Source: CAD feature listing. Evaluate the final solid. Frame: model axes, mm. Coordinates: 2 decimals unless noted, no trailing zeros. Order: outer loops, then holes, each group sorted by start corner. A loop starts at its lowest first (then second) coordinate and runs counter-clockwise, first axis right, second up.
```python
from build123d import *

# Parameters (mm, degrees)
BOSS_EXTRUDE1_DEPTH = 10


with BuildPart() as part:
    # Sketch1 → Boss-Extrude1 (new body)
    with BuildSketch(Plane(origin=(0, 0, 0), x_dir=(1, 0, 0), z_dir=(0, 1, 0))):
        with BuildLine():
            ThreePointArc((2.7, 0), (2.693734095, 0.183838592), (2.674965461, 0.366823913))
            Line((2.674965461, 0.366823913), (1.655161558, 2.133176087))
            ThreePointArc((1.655161558, 2.133176087), (1.35, 2.33826859), (1.019803903, 2.5))
            Line((1.019803903, 2.5), (-1.019803903, 2.5))
            ThreePointArc((-1.019803903, 2.5), (-1.35, 2.33826859), (-1.655161558, 2.133176087))
            Line((-1.655161558, 2.133176087), (-2.674965461, 0.366823913))
            ThreePointArc((-2.674965461, 0.366823913), (-2.7, 0), (-2.674965461, -0.366823913))
            Line((-2.674965461, -0.366823913), (-1.655161558, -2.133176087))
            ThreePointArc((-1.655161558, -2.133176087), (-1.35, -2.33826859), (-1.019803903, -2.5))
            Line((-1.019803903, -2.5), (1.019803903, -2.5))
            ThreePointArc((1.019803903, -2.5), (1.35, -2.33826859), (1.655161558, -2.133176087))
            Line((1.655161558, -2.133176087), (2.674965461, -0.366823913))
            ThreePointArc((2.674965461, -0.366823913), (2.693734095, -0.183838592), (2.7, 0))
        make_face()
    extrude(amount=BOSS_EXTRUDE1_DEPTH)


solid = part.part
```
1. Section query A-A on y = 1.5. Return loops of the section in (x, z), plus the area to 3 significant figures.
Findings:
outline: (-2.67, -0.37) - (-1.66, -2.13) arc R2.7 ccw to (-1.02, -2.5) - (1.02, -2.5) arc R2.7 ccw to (1.66, -2.13) - (2.67, -0.37) arc R2.7 ccw to (2.67, 0.37) - (1.66, 2.13) arc R2.7 ccw to (1.02, 2.5) - (-1.02, 2.5) arc R2.7 ccw to (-1.66, 2.13) - (-2.67, 0.37) arc R2.7 ccw to start
area: 21.3 mm2
2. Ray query, line 1 (X direction, y = 1, z = -1.2); line 2 (Z direction, x = 1.05, y = 2.25); line 3 (Z direction, x = -2.25, y = 9.25). Return the intervals inside material, ascending.
Findings:
line 1: x = -2.19 to 2.19
line 2: z = -2.49 to 2.49
line 3: z = -1.1 to 1.1
3. Section query C-C on x = 2.2. Return loops of the section in (y, z), plus the area to 3 significant figures.
Findings:
outline: (0, -1.19) - (10, -1.19) - (10, 1.19) - (0, 1.19) - close
area: 23.8 mm2
4. Section query B-B on z = -0.9. Return loops of the section in (x, y).
Findings:
outline: (-2.37, 0) - (2.37, 0) - (2.37, 10) - (-2.37, 10) - close
5. Pin query (flat end, axial travel): P1, Ø1.5, axis at x = 1.5, y = 7.5, coming from the -Z side. Return the tip coordinate at first contact, or that it passes through.
Findings:
P1: stops at z = -2.5
